from build123d import *

# Parameters (mm, degrees)
SKETCH1_W           = 68
SKETCH1_H           = 11.5
BOSS_EXTRUDE1_DEPTH = 7.94
SKETCH2_W           = 27.75
SKETCH2_H           = 10
SKETCH2_W_2         = 9.525
SKETCH2_H_2         = 5.5
CUT_EXTRUDE1_DEPTH  = 36.385111276
SKETCH3_W           = 10
SKETCH3_H           = 6.44
CUT_EXTRUDE2_DEPTH  = 69.703028318
SKETCH4_W           = 11
SKETCH4_H           = 2
CUT_EXTRUDE3_DEPTH  = 2.5


with BuildPart() as part:
    # Sketch1 → Boss-Extrude1 (new body)
    with BuildSketch(Plane(origin=(0, 0, 0), x_dir=(1, 0, 0), z_dir=(0, 1, 0))):
        Rectangle(SKETCH1_W, SKETCH1_H)
    extrude(amount=BOSS_EXTRUDE1_DEPTH)

    # Sketch2 → Cut-Extrude1 (cut, through all)
    with BuildSketch(Plane(origin=(0, 7.94, 0), x_dir=(1, 0, 0), z_dir=(0, 1, 0))):
        with Locations((-19.375, 0)):
            Rectangle(SKETCH2_W, SKETCH2_H)
        with Locations((19.375, 0)):
            Rectangle(SKETCH2_W, SKETCH2_H)
        with Locations((0.0125, 0)):
            Rectangle(SKETCH2_W_2, SKETCH2_H_2)
    extrude(amount=-CUT_EXTRUDE1_DEPTH, mode=Mode.SUBTRACT)

    # Sketch3 → Cut-Extrude2 (cut, through all)
    with BuildSketch(Plane.ZY.offset(34)):
        with Locations((0, 3.97)):
            Rectangle(SKETCH3_W, SKETCH3_H)
    extrude(amount=-CUT_EXTRUDE2_DEPTH, mode=Mode.SUBTRACT)

    # Sketch4 → Cut-Extrude3 (cut)
    with BuildSketch(Plane(origin=(0, 7.94, 0), x_dir=(1, 0, 0), z_dir=(0, 1, 0))):
        Rectangle(SKETCH4_W, SKETCH4_H)
    extrude(amount=-CUT_EXTRUDE3_DEPTH, mode=Mode.SUBTRACT)


solid = part.part
Check sheet for the modelled part. Datum: model origin and axes. Units: mm. A direction names the side the tool comes from. Round coordinates to 2 decimals unless told otherwise and drop trailing zeros. Loops run counter-clockwise (first coordinate to the right, second up) from the corner with the lowest first, then second, coordinate; pieces in that order, holes last. Notation, with made-up numbers: M -24,-9 L 10,-9 A19 cw 10,-3 Z; hole C 50.25,-38.75 d4. An arc over 180 degrees is marked long. One line per question, with ' | ' between items. Start each with the question number.
Item 1: Section check C-C (z = -4). Record the boundary of the cut face in (x, y), and give its area (4 significant figures).
Item 2: Gauge pin test, flat ends, axial feed: pin 1 Ø5 at (x, z) = (-9, -3) entering from -Y; pin 2 Ø3 at (x, z) = (-14.5, 3) entering from -Y. Record the tip position at first contact, or that the pin passes through.
Item 3: Release check for a two-part mould opening along Y. For faces 3 (the face through (0, 0, -3)), 4 (the face through (-34, 0.4, 0.1)), 5 (the face through (0, 7.19, -3)) record: released by +Y, released by -Y, zero draft, split by the parting line, or undercut.
Item 4: Section check B-B (x = 20.5). Record the boundary of the cut face in (y, z), and give its area (3 significant figures).
Item 5: Scan lines: probe 1 along X at (y, z) = (7.5, -3.5); probe 2 along Z at (x, y) = (-27.5, 0.75); probe 3 along Y at (x, z) = (1, 4.25). Record each from-to range of solid material in increasing order.
Item 6: Set-up check for faces 1 (the face through (0, 7.19, 3)), 2 (the face through (0, 4, -5.75)): record each of +Z, -Z, +X, -X, +Y, -Y from which the full face is reachable in a straight line by a thin tool's end or side.
Item 7: Section check A-A (y = 2.25). Record the boundary of the cut face in (x, z), and give its area (3 significant figures).
Worked out:
1) outline: M -34,0 L -33.25,0 L -33.25,0.75 L -34,0.75 Z; M -34,7.19 L -33.25,7.19 L -33.25,7.94 L -34,7.94 Z; M -5.5,0 L 5.5,0 L 5.5,0.75 L -5.5,0.75 Z; M -5.5,7.19 L 5.5,7.19 L 5.5,7.94 L -5.5,7.94 Z; M 33.25,0 L 34,0 L 34,0.75 L 33.25,0.75 Z; M 33.25,7.19 L 34,7.19 L 34,7.94 L 33.25,7.94 Z | area: 18.75 mm^2
2) pin 1: y = 0 | pin 2: through
3) face 3: released by -Y | face 4: zero draft | face 5: undercut
4) outline: M 0,-5.75 L 7.94,-5.75 L 7.94,-5 L 0,-5 Z; M 0,5 L 7.94,5 L 7.94,5.75 L 0,5.75 Z | area: 11.9 mm^2
5) probe 1: -34 to -33.25, -5.5 to 5.5, 33.25 to 34 | probe 2: -5.75 to -5, 5 to 5.75 | probe 3: 0 to 0.75, 7.19 to 7.94
6) face 1: +X, -X | face 2: -Z, +X, -X, +Y, -Y
7) outline: M -34,-5.75 L 34,-5.75 L 34,-5 L -34,-5 Z; M -34,5 L 34,5 L 34,5.75 L -34,5.75 Z | area: 102 mm^2
